Part model, mm, in its own coordinate system. Coordinates: 2 decimals unless noted, no trailing zeros. Order: outer loops, then holes, each group sorted by start corner. A loop starts at its lowest first (then second) coordinate and runs counter-clockwise, first axis right, second up.
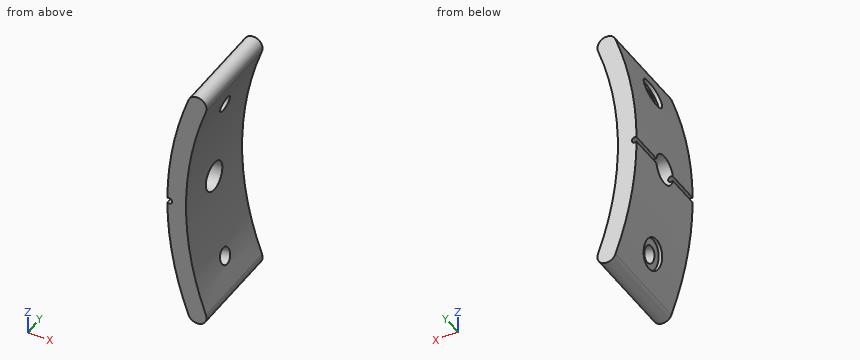
from build123d import *

# Parameters (mm, degrees)
BOSS_EXTRUDE2_DEPTH = 10
SKETCH9_R           = 1.65
CUT_EXTRUDE3_DEPTH  = 10
SKETCH10_R          = 2.95
CUT_EXTRUDE4_DEPTH  = 69.7500001
SKETCH12_R          = 3
CUT_EXTRUDE5_DEPTH  = 2
SKETCH13_R          = 0.6
CUT_EXTRUDE6_DEPTH  = 21.0000001


with BuildPart() as part:
    # Sketch3 → Boss-Extrude2 (new body, symmetric)
    with BuildSketch(Plane(origin=(0, 0, 0), x_dir=(1, 0, 0), z_dir=(0, 1, 0))):
        with BuildLine():
            ThreePointArc((-60.981554588, 22.5), (-65, 0), (-60.981554588, -22.5))
            ThreePointArc((-60.981554588, -22.5), (-62.091599432, -24.908121767), (-64.499721199, -23.798076923))
            ThreePointArc((-64.499721199, -23.798076923), (-68.75, 0), (-64.499721199, 23.798076923))
            ThreePointArc((-64.499721199, 23.798076923), (-62.091599432, 24.908121767), (-60.981554588, 22.5))
        make_face()
    extrude(amount=BOSS_EXTRUDE2_DEPTH, both=True)

    # Sketch9 → Cut-Extrude3 (cut, symmetric)
    with BuildSketch(Plane(origin=(-62.785178709, 0, -16.823237932), x_dir=(0, -1, 0), z_dir=(0.965925826, 0, 0.258819045))):
        Circle(SKETCH9_R)
    cut_extrude3 = extrude(amount=CUT_EXTRUDE3_DEPTH, both=True, mode=Mode.SUBTRACT)

    # Mirror1: Cut-Extrude3 across plane
    add(cut_extrude3.mirror(Plane.XY), mode=Mode.SUBTRACT)

    # Sketch10 → Cut-Extrude4 (cut, through all)
    with BuildSketch(Plane(origin=(0, 0, 0), x_dir=(0, 0, -1), z_dir=(1, 0, 0))):
        Circle(SKETCH10_R)
    extrude(amount=-CUT_EXTRUDE4_DEPTH, mode=Mode.SUBTRACT)

    # Sketch12 → Cut-Extrude5 (cut)
    with BuildSketch(Plane(origin=(-67.61480784, 0, -18.117333157), x_dir=(0, -1, 0), z_dir=(0.965925826, 0, 0.258819045))):
        Circle(SKETCH12_R)
    cut_extrude5 = extrude(amount=CUT_EXTRUDE5_DEPTH, mode=Mode.SUBTRACT)

    # Mirror2: Cut-Extrude5 across plane
    add(cut_extrude5.mirror(Plane.XY), mode=Mode.SUBTRACT)

    # Sketch13 → Cut-Extrude6 (cut, through all)
    with BuildSketch(Plane(origin=(0, 10, 0), x_dir=(1, 0, 0), z_dir=(0, 1, 0))):
        with Locations((-68.4, 0)):
            Circle(SKETCH13_R)
    extrude(amount=-CUT_EXTRUDE6_DEPTH, mode=Mode.SUBTRACT)


solid = part.part
Q1. Cut at B-B on y = 0. Count the separate pieces of the cut face and the enclosed holes in it, and give its area (3 significant figures).
Results list:
separate pieces: 4
enclosed holes: 0
area: 138 mm2
Q2. Wall check: line 1 along Y through (x, z) = (-67.55, 0); line 2 along Z through (x, y) = (-66.5, 2.5); line 3 along Z through (x, y) = (-65.7, 0). Give the ranges that are in metal, low to high.
Results list:
line 1: y = -10 to -2.95, 2.95 to 10
line 2: z = -16.1 to -1.57, 1.57 to 16.1
line 3: z = -15.9 to -2.95, 2.95 to 15.9
Q3. Cut at C-C on y = -5.75. Write the cut outline in (x, z) (3 decimals), and give its area (3 significant figures).
Results list:
outline: (-68.748, -0.489) arc R68.75 ccw to (-64.5, -23.798) arc R1.875 ccw to (-60.982, -22.5) arc R65 cw to (-60.982, 22.5) arc R1.875 ccw to (-64.5, 23.798) arc R68.75 ccw to (-68.748, 0.489) arc R0.6 cw (long way) to start
area: 187 mm2
Q4. Cut at D-D on y = -2.25. Write the cut outline in (x, z) (3 decimals), and give its area (3 significant figures).
Results list:
outline: (-68.724, -1.908) arc R68.75 ccw to (-66.893, -15.87) - (-66.197, -15.683) - (-65.169, -19.516) - (-65.866, -19.703) arc R68.75 ccw to (-64.5, -23.798) arc R1.875 ccw to (-60.982, -22.5) arc R65 cw to (-64.972, -1.908) - close; (-68.724, 1.908) - (-64.972, 1.908) arc R65 cw to (-60.982, 22.5) arc R1.875 ccw to (-64.5, 23.798) arc R68.75 ccw to (-65.866, 19.703) - (-65.169, 19.516) - (-66.197, 15.683) - (-66.893, 15.87) arc R68.75 ccw to start
area: 168 mm2
Q5. Cut at A-A on z = 0. Write the cut outline in (x, y), and give its area (3 significant figures).
Results list:
outline: (-67.8, -10) - (-65, -10) - (-65, -2.95) - (-67.8, -2.95) - close; (-67.8, 2.95) - (-65, 2.95) - (-65, 10) - (-67.8, 10) - close
area: 39.5 mm2
Q6. Pin check, flat tips, straight feed: pin 1 Ø4 at (y, z) = (3, -9.5) entering from +X; pin 2 Ø8 at (y, z) = (-1.5, 3) entering from +X; pin 3 Ø5.5 at (y, z) = (0, 0) entering from -X; pin 4 Ø2 at (x, y) = (-65, 7) entering from +Z. Stop position of each tip, or through.
Results list:
pin 1: stops at x = -63.97
pin 2: stops at x = -64.62
pin 3: passes through
pin 4: stops at z = 24.54
